Design review of the part shown in the three views and the two pictorial views. Dimensions are in mm from the part's minimum x, y and z. A direction names the side the tool comes from. Coordinates: 2 decimals unless noted, no trailing zeros. Loops run counter-clockwise (first coordinate to the right, second up) from the corner with the lowest first, then second, coordinate; pieces in that order, holes last. Notation, with made-up numbers: (-37, 88.25) -> (-30, 88.25) arc R19 cw to (-30, 94.25) -> close; hole circle Ø1 at (38, -21). An arc over 180 degrees is marked (long way). Answer in a Markdown table with one row per item.
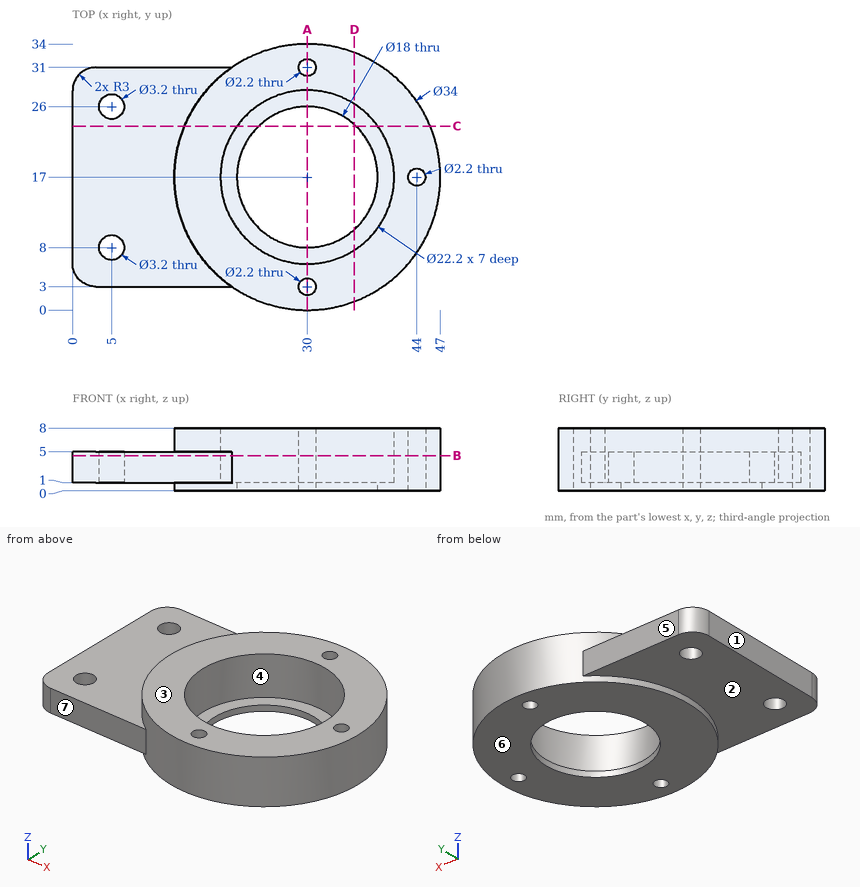
(1) Draft analysis for pull direction Z (two halves, no side actions). For the marked faces 1, 2 and 3, state which applies: pulls with the +Z half, pulls with the -Z half, needs draft (parallel to the pull), parting line crosses it, or undercut.
Evaluation:
| item | result |
|---|---|
| face 1 | needs draft |
| face 2 | pulls with the -Z half |
| face 3 | pulls with the +Z half |
(2) Take a section at B-B on z = 4.5. Give the boundary of the cut face in (x, y), and give its area (3 significant figures).
Evaluation:
| item | result |
|---|---|
| outline | (0, 6) arc R3 ccw to (3, 3) -> (20.36, 3) arc R17 ccw (long way) to (20.36, 31) -> (3, 31) arc R3 ccw to (0, 28) -> close; hole circle Ø3.2 at (5, 8); hole circle Ø3.2 at (5, 26); hole circle Ø22.2 at (30, 17); hole circle Ø2.2 at (30, 3); hole circle Ø2.2 at (30, 31); hole circle Ø2.2 at (44, 17) |
| area | 915 mm² |
(3) For pin 1 (4 mm diameter, centred on x = 5.5, y = 28.5, fed in from +Z); pin 2 (3 mm diameter, centred on x = 14, z = 2.5, fed in from -Y); pin 3 (2 mm diameter, centred on x = 21, y = 21, fed in from +Z), all flat-tipped, find the tip position at first contact; note any pin that passes through.
Evaluation:
| item | result |
|---|---|
| pin 1 | stops at z = 5 |
| pin 2 | stops at y = 3 |
| pin 3 | stops at z = 1 |
(4) Take a section at A-A on x = 30. Give the boundary of the cut face in (y, z), and give its area (3 significant figures).
Evaluation:
| item | result |
|---|---|
| outline | (0, 0) -> (1.9, 0) -> (1.9, 8) -> (0, 8) -> close; (4.1, 0) -> (8, 0) -> (8, 1) -> (5.9, 1) -> (5.9, 8) -> (4.1, 8) -> close; (26, 0) -> (29.9, 0) -> (29.9, 8) -> (28.1, 8) -> (28.1, 1) -> (26, 1) -> close; (32.1, 0) -> (34, 0) -> (34, 8) -> (32.1, 8) -> close |
| area | 63.4 mm² |
(5) To check wall thickness, follow probe 1 along Y at (x, z) = (31, 6.75); probe 2 along Y at (x, z) = (30.5, 5.5); probe 3 along X at (y, z) = (17.5, 5.5). State the ranges of each line that lie inside material, in increasing order.
Evaluation:
| item | result |
|---|---|
| probe 1 | y = 0.03 to 2.54, 3.46 to 5.95, 28.05 to 30.54, 31.46 to 33.97 |
| probe 2 | y = 0.01 to 2.02, 3.98 to 5.91, 28.09 to 30.02, 31.98 to 33.99 |
| probe 3 | x = 13.01 to 18.91, 41.09 to 43.02, 44.98 to 46.99 |
(6) Take a section at D-D on x = 36. Give the boundary of the cut face in (y, z).
Evaluation:
| item | result |
|---|---|
| outline | (1.09, 0) -> (10.29, 0) -> (10.29, 1) -> (7.66, 1) -> (7.66, 8) -> (1.09, 8) -> close; (23.71, 0) -> (32.91, 0) -> (32.91, 8) -> (26.34, 8) -> (26.34, 1) -> (23.71, 1) -> close |
(7) Take a section at C-C on y = 23.5. Give the boundary of the cut face in (x, z).
Evaluation:
| item | result |
|---|---|
| outline | (0, 1) -> (14.29, 1) -> (14.29, 0) -> (23.78, 0) -> (23.78, 1) -> (21, 1) -> (21, 8) -> (14.29, 8) -> (14.29, 5) -> (0, 5) -> close; (36.22, 0) -> (45.71, 0) -> (45.71, 8) -> (39, 8) -> (39, 1) -> (36.22, 1) -> close |
(8) Tool access review of the marked faces 4, 5, 6 and 7: name each direction out of +Z, -Z, +X, -X, +Y, -Y from which nothing blocks a thin tool from reaching the whole face with its end or side.
Evaluation:
| item | result |
|---|---|
| face 4 | +Z |
| face 5 | +Z, -Z, -X, +Y |
| face 6 | -Z, +X, -X, +Y, -Y |
| face 7 | +Z, -Z, -X, -Y |
